```python
from build123d import *

# Parameters (mm, degrees)
SKETCH1_R          = 1.5
SKETCH1_R_2        = 6
SKETCH1_R_3        = 1.55
BASE_FLANGE1_DEPTH = 1


# Sheet-metal steps are written as plain solids
with BuildPart() as part:
    # Sketch1 → Base-Flange1 (new body)
    with BuildSketch(Plane(origin=(0, 0, 0), x_dir=(0, 0, -1), z_dir=(1, 0, 0))):
        with BuildLine():
            Line((15.298384889, 9.287443872), (23.016301233, 1.688033071))
            ThreePointArc((23.016301233, 1.688033071), (25.224073123, -1.574984432), (26.00015012, -5.437528209))
            Line((26.00015012, -5.437528209), (26.00015012, -12.25))
            ThreePointArc((26.00015012, -12.25), (22.75007506, -15.50007506), (19.5, -12.25))
            Line((19.5, -12.25), (19.5, -4.25))
            ThreePointArc((19.5, -4.25), (18.5, -3.25), (17.5, -4.25))
            Line((17.5, -4.25), (17.583796073, -15.080985895))
            ThreePointArc((17.583796073, -15.080985895), (16.837624745, -18.949418172), (14.655163154, -22.229418377))
            Line((14.655163154, -22.229418377), (9.838018154, -27.046563377))
            ThreePointArc((9.838018154, -27.046563377), (5.241717926, -27.046563377), (5.241717926, -22.450263149))
            Line((5.241717926, -22.450263149), (10.898572175, -16.793408899))
            ThreePointArc((10.898572175, -16.793408899), (10.898572175, -15.379195337), (9.484358613, -15.379195337))
            Line((9.484358613, -15.379195337), (1.884947812, -23.097111681))
            ThreePointArc((1.884947812, -23.097111681), (-1.378069691, -25.304883571), (-5.240613468, -26.080960568))
            Line((-5.240613468, -26.080960568), (-12.053085259, -26.080960568))
            ThreePointArc((-12.053085259, -26.080960568), (-15.303160319, -22.830885508), (-12.053085259, -19.580810448))
            Line((-12.053085259, -19.580810448), (-4.053085259, -19.580810448))
            ThreePointArc((-4.053085259, -19.580810448), (-3.053085259, -18.580810448), (-4.053085259, -17.580810448))
            Line((-4.053085259, -17.580810448), (-14.884071154, -17.664606521))
            ThreePointArc((-14.884071154, -17.664606521), (-18.752503431, -16.918435193), (-22.032503636, -14.735973602))
            Line((-22.032503636, -14.735973602), (-26.849648636, -9.918828602))
            ThreePointArc((-26.849648636, -9.918828602), (-26.849648636, -5.322528374), (-22.253348408, -5.322528374))
            Line((-22.253348408, -5.322528374), (-16.596494158, -10.979382623))
            ThreePointArc((-16.596494158, -10.979382623), (-15.182280596, -10.979382623), (-15.182280596, -9.565169061))
            Line((-15.182280596, -9.565169061), (-22.90019694, -1.96575826))
            ThreePointArc((-22.90019694, -1.96575826), (-25.10796883, 1.297259243), (-25.884045827, 5.15980302))
            Line((-25.884045827, 5.15980302), (-25.884045827, 11.972274811))
            ThreePointArc((-25.884045827, 11.972274811), (-22.633970767, 15.222349871), (-19.383895707, 11.972274811))
            Line((-19.383895707, 11.972274811), (-19.383895707, 3.972274811))
            ThreePointArc((-19.383895707, 3.972274811), (-18.383895707, 2.964508185), (-17.383895707, 3.972274811))
            Line((-17.383895707, 3.972274811), (-17.46769178, 14.803260706))
            ThreePointArc((-17.46769178, 14.803260706), (-16.721520452, 18.671692983), (-14.539058861, 21.951693188))
            Line((-14.539058861, 21.951693188), (-9.721913861, 26.768838188))
            ThreePointArc((-9.721913861, 26.768838188), (-5.125613633, 26.768838188), (-5.125613633, 22.17253796))
            Line((-5.125613633, 22.17253796), (-10.782467882, 16.51568371))
            ThreePointArc((-10.782467882, 16.51568371), (-10.787959717, 15.095978314), (-9.36825432, 15.101470148))
            Line((-9.36825432, 15.101470148), (-1.768843519, 22.819386492))
            ThreePointArc((-1.768843519, 22.819386492), (1.494173984, 25.027158382), (5.356717761, 25.803235379))
            Line((5.356717761, 25.803235379), (12.169189552, 25.803235379))
            ThreePointArc((12.169189552, 25.803235379), (15.419264612, 22.553160319), (12.169189552, 19.303085259))
            Line((12.169189552, 19.303085259), (4.169189552, 19.303085259))
            ThreePointArc((4.169189552, 19.303085259), (3.161422926, 18.303085259), (4.169189552, 17.303085259))
            Line((4.169189552, 17.303085259), (15.000175447, 17.386881332))
            ThreePointArc((15.000175447, 17.386881332), (18.868607724, 16.640710004), (22.148607929, 14.458248413))
            Line((22.148607929, 14.458248413), (26.965752929, 9.641103413))
            ThreePointArc((26.965752929, 9.641103413), (26.965752929, 5.044803185), (22.369452701, 5.044803185))
            Line((22.369452701, 5.044803185), (16.712598451, 10.701657434))
            ThreePointArc((16.712598451, 10.701657434), (15.298384889, 10.701657434), (15.298384889, 9.287443872))
        make_face()
        with Locations((22.75007506, -12.25)):
            Circle(SKETCH1_R, mode=Mode.SUBTRACT)
        with Locations((7.53986804, -24.748413263)):
            Circle(SKETCH1_R, mode=Mode.SUBTRACT)
        with Locations((-12.053085259, -22.830885508)):
            Circle(SKETCH1_R, mode=Mode.SUBTRACT)
        with Locations((-24.551498522, -7.620678488)):
            Circle(SKETCH1_R, mode=Mode.SUBTRACT)
        with Locations((-22.633970767, 11.972274811)):
            Circle(SKETCH1_R, mode=Mode.SUBTRACT)
        with Locations((-7.423763747, 24.470688074)):
            Circle(SKETCH1_R, mode=Mode.SUBTRACT)
        with Locations((12.169189552, 22.553160319)):
            Circle(SKETCH1_R, mode=Mode.SUBTRACT)
        with Locations((24.667602815, 7.342953299)):
            Circle(SKETCH1_R, mode=Mode.SUBTRACT)
        Circle(SKETCH1_R_2, mode=Mode.SUBTRACT)
        with Locations((0, 10)):
            Circle(SKETCH1_R_3, mode=Mode.SUBTRACT)
        with Locations((8.660254038, -5)):
            Circle(SKETCH1_R_3, mode=Mode.SUBTRACT)
        with Locations((-8.660254038, -5)):
            Circle(SKETCH1_R_3, mode=Mode.SUBTRACT)
    extrude(amount=-BASE_FLANGE1_DEPTH)


solid = part.part
```
Geometry: final body of the model. Coordinates: model frame, mm. A direction names the side the tool comes from. Give positions to 0.01 mm unless a question says otherwise; leave off trailing zeros. Write each loop counter-clockwise with the first axis right and the second up, starting at its lowest first coordinate (ties: lowest second). Pieces come first, ordered by that corner, then holes.
1. Draft query along Y for faces 4 (the flat face through (-0.49, -12.36, 24.41)), 5 (the flat face through (-0.493, 12.083, -24.523)), 6 (the cylindrical face through (-0.49, 1.25, 25.09)). Return one class per face: released by +Y, released by -Y, zero draft, split by the parting line, or undercut.
2. Line query: probe 1 along Z at (x, y) = (-0.25, 12.5); probe 2 along Y at (x, z) = (-0.3, 0); probe 3 along Z at (x, y) = (-0.35, 9). Output: solid intervals per line, ascending.
3. Section query A-A, the plane z = -18.5. Return loops of the section in (x, y), then the cut area to 3 significant figures.
4. Section query D-D, the plane z = 0. Return loops of the section in (x, y), then the cut area to 3 significant figures.
5. Reachability of faces 1 (the cylindrical face through (-0.493, 25.006, -1.443)), 2 (the flat face through (-0.493, -5.819, 18.987)), 3 (the cylindrical face through (-0.49, -1.52, -25.2)) from +Z, -Z, +X, -X, +Y, -Y: full face, straight path, thin tool, end or side. Return the list, or none.
6. Section query C-C, the plane y = 20. Return loops of the section in (x, z), then the cut area to 3 significant figures.
7. Section query B-B, the plane z = -8. Return loops of the section in (x, y), then the cut area to 3 significant figures.
8. Pin query (flat end, axial travel): P1, Ø0.5, axis at x = -0.5, z = 9, coming from the +Y side; P2, Ø5, axis at y = -24.75, z = -7.54, coming from the -X side; P3, Ø1.8, axis at y = -22.83, z = 12.05, coming from the -X side; P4, Ø0.5, axis at x = -0.5, y = -9, coming from the +Z side. Return the tip coordinate at first contact, or that it passes through.
Computed:
1. face 4: released by -Y
1. face 5: released by +Y
1. face 6: undercut
2. probe 1: z = -24.11 to 17.45, 19.43 to 21.23, 24.04 to 25.84
2. probe 2: y = -24.6 to -6, 6 to 8.45, 11.55 to 24.25
2. probe 3: z = -27.46 to -18.41, -15.59 to -1.18, 1.18 to 17.42, 19.38 to 25.88
3. outline: (-1, -3.25) - (0, -3.25) - (0, 6.13) - (-1, 6.13) - close; (-1, 8.91) - (0, 8.91) - (0, 16.78) - (-1, 16.78) - close
3. area: 17.3 mm2
4. outline: (-1, -24.6) - (0, -24.6) - (0, -6) - (-1, -6) - close; (-1, 6) - (0, 6) - (0, 8.45) - (-1, 8.45) - close; (-1, 11.55) - (0, 11.55) - (0, 24.25) - (-1, 24.25) - close
4. area: 33.7 mm2
5. face 1: +X, -X, +Y
5. face 2: +X, -X
5. face 3: -Z, +X, -X
6. outline: (-1, -14.18) - (0, -14.18) - (0, 4.54) - (-1, 4.54) - close; (-1, 7.3) - (0, 7.3) - (0, 16.06) - (-1, 16.06) - close
6. area: 27.5 mm2
7. outline: (-1, -27.97) - (0, -27.97) - (0, -26.18) - (-1, -26.18) - close; (-1, -23.32) - (0, -23.32) - (0, -19.69) - (-1, -19.69) - close; (-1, -16.89) - (0, -16.89) - (0, -6.4) - (-1, -6.4) - close; (-1, -3.6) - (0, -3.6) - (0, 17.33) - (-1, 17.33) - close; (-1, 19.3) - (0, 19.3) - (0, 25.8) - (-1, 25.8) - close
7. area: 43.3 mm2
8. P1: stops at y = 27.44
8. P2: stops at x = -1
8. P3: passes through
8. P4: stops at z = 27.6
